from build123d import *

# Parameters (mm, degrees)
CROQUIS1_W                                 = 340
CROQUIS1_H                                 = 42
CROQUIS1_R                                 = 2.5
CROQUIS1_R_2                               = 1.5
SALIENTE_EXTRUIR1_DEPTH                    = 3
CROQUIS2_W                                 = 15
CROQUIS2_H                                 = 4
CORTAR_EXTRUIR1_DEPTH                      = 172.31841699
SIMETR_A1_AT_THE_SECOND_PLANE_COPY_1_SKE_W = 15
SIMETR_A1_AT_THE_SECOND_PLANE_COPY_1_SKE_H = 4
SIMETR_A1_AT_THE_SECOND_PLANE_COPY_1_DEPTH = 172.31841699
REDONDEO1_R                                = 2
CROQUIS3_W                                 = 261
CROQUIS3_H                                 = 11.873622062
CORTAR_EXTRUIR2_DEPTH                      = 172.31841699
CROQUIS7_W                                 = 13
CROQUIS7_H                                 = 4
SALIENTE_EXTRUIR3_DEPTH                    = 3
REDONDEO2_R                                = 2


with BuildPart() as part:
    # Croquis1 → Saliente-Extruir1 (new body)
    with BuildSketch(Plane.XY):
        Rectangle(CROQUIS1_W, CROQUIS1_H)
        with Locations((160, 4)):
            Circle(CROQUIS1_R, mode=Mode.SUBTRACT)
        with Locations((95, 6.5)):
            Circle(CROQUIS1_R_2, mode=Mode.SUBTRACT)
        with Locations((125, -14)):
            Circle(CROQUIS1_R_2, mode=Mode.SUBTRACT)
        with Locations((95, -14)):
            Circle(CROQUIS1_R_2, mode=Mode.SUBTRACT)
        with Locations((125, 6.5)):
            Circle(CROQUIS1_R_2, mode=Mode.SUBTRACT)
        with Locations((-113, -14)):
            Circle(CROQUIS1_R_2, mode=Mode.SUBTRACT)
        with Locations((-104, 6.5)):
            Circle(CROQUIS1_R_2, mode=Mode.SUBTRACT)
        with Locations((-95, -14)):
            Circle(CROQUIS1_R_2, mode=Mode.SUBTRACT)
        with Locations((-155, 4)):
            Circle(CROQUIS1_R, mode=Mode.SUBTRACT)
        with Locations((82, -5)):
            Circle(CROQUIS1_R_2, mode=Mode.SUBTRACT)
        with Locations((60, -5)):
            Circle(CROQUIS1_R_2, mode=Mode.SUBTRACT)
    extrude(amount=SALIENTE_EXTRUIR1_DEPTH)

    # Croquis2 → Cortar-Extruir1 (cut, through all)
    with BuildSketch(Plane.XY.offset(3)):
        with Locations((-162.5, -19)):
            Rectangle(CROQUIS2_W, CROQUIS2_H)
    cortar_extruir1 = extrude(amount=-CORTAR_EXTRUIR1_DEPTH, mode=Mode.SUBTRACT)

    # Simetría1: Cortar-Extruir1 across plane
    add(cortar_extruir1.mirror(Plane.ZX), mode=Mode.SUBTRACT)

    # Simetría1 at the second plane: Cortar-Extruir1 across plane
    add(cortar_extruir1.mirror(Plane(origin=(0, 0, 0), x_dir=(0, 0, 1), z_dir=(1, 0, 0))), mode=Mode.SUBTRACT)

    # Simetría1 at the second plane copy 1 ske → Simetría1 at the second plane copy 1 (cut, through all)
    with BuildSketch(Plane(origin=(0, 0, 3), x_dir=(-1, 0, 0), z_dir=(0, 0, 1))):
        with Locations((-162.5, -19)):
            Rectangle(SIMETR_A1_AT_THE_SECOND_PLANE_COPY_1_SKE_W, SIMETR_A1_AT_THE_SECOND_PLANE_COPY_1_SKE_H)
    extrude(amount=-SIMETR_A1_AT_THE_SECOND_PLANE_COPY_1_DEPTH, mode=Mode.SUBTRACT)

    # Redondeo1
    redondeo1_edges = [part.edges().sort_by_distance(p)[0] for p in [
        (170, 17, 1.5),
        (155, 21, 1.5),
        (-170, -17, 1.5),
        (-155, -21, 1.5),
        (170, -17, 1.5),
        (155, -21, 1.5),
        (-170, 17, 1.5),
    ]]
    fillet(redondeo1_edges, radius=REDONDEO1_R)

    # Croquis3 → Cortar-Extruir2 (cut, through all)
    with BuildSketch(Plane.XY.offset(3)):
        with Locations((-20.5, 22.936811031)):
            Rectangle(CROQUIS3_W, CROQUIS3_H)
    extrude(amount=-CORTAR_EXTRUIR2_DEPTH, mode=Mode.SUBTRACT)

    # Croquis7 → Saliente-Extruir3 (add)
    with BuildSketch(Plane.XY.offset(3)):
        with Locations((-157.5, 19)):
            Rectangle(CROQUIS7_W, CROQUIS7_H)
    extrude(amount=-SALIENTE_EXTRUIR3_DEPTH)

    # Redondeo2
    redondeo2_edges = [part.edges().sort_by_distance(p)[0] for p in [
        (110, 21, 1.5),
        (-151, 21, 1.5),
        (-164, 21, 1.5),
    ]]
    fillet(redondeo2_edges, radius=REDONDEO2_R)


solid = part.part
Design review of the part built by this model. Coordinates are the model's own, in mm. Coordinates: 2 decimals unless noted, no trailing zeros. Order: outer loops, then holes, each group sorted by start corner. A loop starts at its lowest first (then second) coordinate and runs counter-clockwise, first axis right, second up. Notation, with made-up numbers: (89.5, -1.75) -> (141.5, -1.75) arc R23 ccw to (141.5, 12.25) -> close; hole circle Ø5 at (39, 64.5). An arc over 180 degrees is marked (long way). Use one line per item in the form item = value. Start each with the question number.
(1) For probe 1 along X at (y, z) = (3.5, 1.95); probe 2 along X at (y, z) = (7, 2.35); probe 3 along Y at (x, z) = (-104, 2.2), list the stretches that pass through material, from the lowest coordinate up.
(2) Add section B-B on x = -26. State the section outline as (y, z) points.
(3) Insertion check: pin 1 (0.6 mm diameter, centred on y = 18, z = 1.5, fed in from -X); pin 2 (1 mm diameter, centred on y = -18, z = 1, fed in from -X); pin 3 (0.9 mm diameter, centred on x = 31.5, z = 2, fed in from +Y). Each pin has a flat end and moves straight along its axis. Give the tip position at first contact, or say it passes through.
(4) Add section A-A on z = 0.5. Give the number of separate pieces and of enclosed holes in the cut face, plus the area to 3 significant figures.
Answer block:
q1.probe_1 = -170 to -157.45, -152.55 to 157.55, 162.45 to 170
q1.probe_2 = -170 to -105.41, -102.59 to 93.59, 96.41 to 123.59, 126.41 to 170
q1.probe_3 = -21 to 5, 8 to 17
q2.outline = (-21, 0) -> (17, 0) -> (17, 3) -> (-21, 3) -> close
q3.pin_1 = -164
q3.pin_2 = -155
q3.pin_3 = 17
q4.separate_pieces = 1
q4.enclosed_holes = 11
q4.area = 12,900 mm²
